Autodesk Inventor part; units mm, degrees
ref_plane "YZ Plane" through (0, 0, 0) normal (1, 0, 0) x (0, 1, 0)
ref_plane "XZ Plane" through (0, 0, 0) normal (0, 1, 0) x (-1, 0, 0)
ref_plane "XY Plane" through (0, 0, 0) normal (0, 0, 1) x (1, 0, 0)
sketch "Sketch1" plane through (0, 0, 0) normal (0, 1, 0) x (-1, 0, 0)
  point P0 (0, 0)
sketch "Sketch2" plane through (0, 0, 0) normal (0, 1, 0) x (-1, 0, 0)
  line L0 (0, 0) -> (-51, 0)
  line L1 (-51, 0) -> (-51, -45)
  line L2 (-51, -45) -> (0, -45)
  line L3 (0, 0) -> (0, -45)
  line L4 (0, -45) -> (0, -22.5)
  circle A0 centre (-21.5, -22.5) radius 12.5
  dimension "d0" = 51
  dimension "d1" = 45
  dimension "d6" = 25
extrude "Extrusion1" add sketch "Sketch2" along normal blind 11
sketch "Sketch3" plane through (0, 11, 0) normal (0, 1, 0) x (1, 0, 0)
  line L0 (0, 45) -> (0, 0)
  line L1 (51, 0) -> (51, 45)
  line L2 (0, 0) -> (51, 0)
  line L3 (51, 0) -> (51, 45)
  line L4 (51, 45) -> (0, 45)
  line L5 (0, 45) -> (0, 0)
extrude "Extrusion2" add sketch "Sketch3" along normal blind 7
sketch "Sketch4" plane through (0, 18, 0) normal (0, 1, 0) x (1, 0, 0)
  line L0 (0, 45) -> (0, 0)
  line L1 (0, 0) -> (51, 0)
  line L2 (3, 14) -> (3, 31)
  line L3 (3, 22.5) -> (3, 20.3)
  line L4 (3, 20.3) -> (3, 24.7)
  line L5 (17.5, 19.5) -> (3, 20.3)
  line L6 (3, 24.7) -> (17.5, 25.5)
  line L7 (17.5, 25.5) -> (17.5, 31.5)
  line L8 (17.5, 31.5) -> (21.5, 31.5)
  line L9 (21.5, 31.5) -> (21.5, 26.5)
  line L10 (17.5, 19.5) -> (17.5, 13.5)
  line L11 (17.5, 13.5) -> (21.5, 13.5)
  line L12 (21.5, 13.5) -> (21.5, 18.5)
  line L13 (38.5, 22.5) -> (38.5, 20.3)
  line L14 (38.5, 20.3) -> (38.5, 24.7)
  line L15 (38.5, 24.7) -> (21.5, 26.5)
  line L16 (38.5, 20.3) -> (21.5, 18.5)
  dimension "d13" = 17
  dimension "d14" = 2.2
  dimension "d15" = 4.4
  dimension "d18" = 6
  dimension "d19" = 6
  dimension "d20" = 4
  dimension "d21" = 5
  dimension "d23" = 6
  dimension "d24" = 4
  dimension "d25" = 5
  dimension "d26" = 2.2
  dimension "d27" = 4.4
extrude "Extrusion3" cut sketch "Sketch4" against normal blind 4
properties part number "CameraOverServo"
The listing builds one solid part. Answer for the finished solid, in the listing's coordinates (mm). A direction names the side the tool comes from. Give positions to 0.01 mm unless a question says otherwise; leave off trailing zeros. Loops run counter-clockwise (first coordinate to the right, second up) from the corner with the lowest first, then second, coordinate; pieces in that order, holes last. Notation, with made-up numbers: M 36,19.5 L 74,19.5 A28 ccw 74,57.5 Z; hole C 8,-6.75 d3. An arc over 180 degrees is marked long. One line per item, written item: value.
Q1. A cutting plane is placed at A-A on y = 14.75. Determine the outline of the cut face in (x, z).
Working result:
outline: M 0,-45 L 51,-45 L 51,0 L 0,0 Z; hole M 3,-24.7 L 17.5,-25.5 L 17.5,-31.5 L 21.5,-31.5 L 21.5,-26.5 L 38.5,-24.7 L 38.5,-20.3 L 21.5,-18.5 L 21.5,-13.5 L 17.5,-13.5 L 17.5,-19.5 L 3,-20.3 Z
Q2. A flat-ended cylindrical pin translates along its axis: P1, Ø22.5, axis at x = 21.5, z = -22.5, coming from the -Y side. Find the tip coordinate at first contact, or state that the pin passes through.
Working result:
P1: stops at y = 11
Q3. For faces 4 (the face through (31.42, 5.423, -14.894)), 5 (the face through (17.5, 16, -28)), 6 (the face through (25, 18, -28)), determine the directions among +Z, -Z, +X, -X, +Y, -Y from which every point of the face is accessible in a straight line to the end or side of a thin tool.
Working result:
face 4: -Y
face 5: +Y
face 6: +Z, -Z, +X, -X, +Y
Q4. A cutting plane is placed at B-B on z = -22.5. Determine the outline of the cut face in (x, y), then the cut area to 3 significant figures.
Working result:
outline: M 0,0 L 9,0 L 9,11 L 34,11 L 34,0 L 51,0 L 51,18 L 38.5,18 L 38.5,14 L 3,14 L 3,18 L 0,18 Z
area: 501 mm^2
Q5. Determine the mould class of faces 1 (the face through (30.119, 16.028, -25.587)), 2 (the face through (37, 0, -22)), 3 (the face through (51, 9, -22)) for opening direction X: +X half, -X half, draft (parallel to the pull), parting line (faces both ways), or undercut.
Working result:
face 1: undercut
face 2: draft
face 3: +X half
Q6. A cutting plane is placed at C-C on x = 14.5. Determine the outline of the cut face in (y, z).
Working result:
outline: M 0,-45 L 18,-45 L 18,-25.33 L 14,-25.33 L 14,-19.67 L 18,-19.67 L 18,0 L 0,0 L 0,-12.14 L 11,-12.14 L 11,-32.86 L 0,-32.86 Z
Q7. Find the intervals of material crossed by line 1 (Z direction, x = 21.5, y = 7.75); line 2 (Y direction, x = 31, z = -24); line 3 (Z direction, x = 18.5, y = 9), in increasing order. Write a range as from..to.
Working result:
line 1: z = -45..-35, -10..0
line 2: y = 11..14
line 3: z = -45..-34.63, -10.37..0
Q8. A cutting plane is placed at D-D on y = 7.75. Determine the outline of the cut face in (x, z), then the cut area to 3 significant figures.
Working result:
outline: M 0,-45 L 51,-45 L 51,0 L 0,0 Z; hole C 21.5,-22.5 d25
area: 1,800 mm^2
